```python
from build123d import *

# Parameters (mm, degrees)
F0_W     = 15
F0_H     = 15
F1_DEPTH = 8.6


with BuildPart() as f1:
    # F0 (on Top) → F1 (new body)
    with BuildSketch(Plane.XY):
        with Locations((-7.5, 13.519098)):
            Rectangle(F0_W, F0_H)
    extrude(amount=F1_DEPTH)

    # F2 (on face) → F3 (revolve, cut)
    with BuildSketch(Plane.XY.offset(8.6)):
        with BuildLine():
            Line((-7.5, 8.752942), (-7.5, 18.752942))
            ThreePointArc((-7.5, 18.752942), (-12.5, 13.752942), (-7.5, 8.752942))
        make_face()
    revolve(axis=Axis((-7.5, 13.752942, 8.6), (0, -1, 0)), mode=Mode.SUBTRACT)


solid = f1.part
```
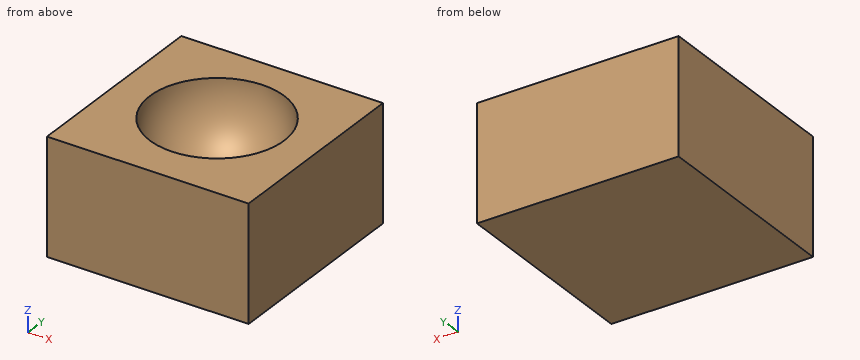
CAD build for the part. Positions are in the model's coordinates, mm. Coordinates: 2 decimals unless noted, no trailing zeros. Write each loop counter-clockwise with the first axis right and the second up, starting at its lowest first coordinate (ties: lowest second). Pieces come first, ordered by that corner, then holes. Notation, with made-up numbers: (82, 74) -> (99, 74) arc R25 ccw to (99, 90) -> close; hole circle Ø8 at (40, 54.25). An arc over 180 degrees is marked (long way). Use CSV: the item, a comma, the result in double quotes. Start each with the question number.
Item 1: Wall check: probe 1 along X at (y, z) = (13.75, 6.75); probe 2 along Y at (x, z) = (-7.5, 4.25); probe 3 along X at (y, z) = (15.5, 5). Give the ranges that are in metal, low to high.
Item 2: Band-saw the part on B-B, the plane x = -9. Write the cut outline in (y, z), plus the area to 3 significant figures.
Item 3: Band-saw the part on A-A, the plane z = 5.5. Write the cut outline in (x, y), plus the area to 3 significant figures.
Item 4: Band-saw the part on D-D, the plane z = 7. Write the cut outline in (x, y).
Item 5: Band-saw the part on C-C, the plane y = 10.25. Write the cut outline in (x, z).
Response values:
1,probe 1,"x = -15 to -12.15, -2.85 to 0"
1,probe 2,"y = 6.02 to 11.29, 16.22 to 21.02"
1,probe 3,"x = -15 to -10.5, -4.5 to 0"
2,outline,"(6.02, 0) -> (21.02, 0) -> (21.02, 8.6) -> (18.52, 8.6) arc R4.77 cw to (8.98, 8.6) -> (6.02, 8.6) -> close"
2,area,"93.3 mm2"
3,outline,"(-15, 6.02) -> (0, 6.02) -> (0, 21.02) -> (-15, 21.02) -> close; hole circle Ø7.85 at (-7.5, 13.75)"
3,area,"177 mm2"
4,outline,"(-15, 6.02) -> (0, 6.02) -> (0, 21.02) -> (-15, 21.02) -> close; hole circle Ø9.47 at (-7.5, 13.75)"
5,outline,"(-15, 0) -> (0, 0) -> (0, 8.6) -> (-3.93, 8.6) arc R3.57 cw to (-11.07, 8.6) -> (-15, 8.6) -> close"
